from build123d import *
from OCP.BRepFilletAPI import BRepFilletAPI_MakeChamfer

# Parameters (mm, degrees)
SKETCH1_W           = 2.1
SKETCH1_H           = 6.25
BOSS_EXTRUDE1_DEPTH = 39
DRAFT1_ANGLE        = -30
DRAFT2_ANGLE        = -30
CHAMFER1_SIZE       = 0.1
CHAMFER2_SIZE       = 0.273205081
CHAMFER2_SIZE_2     = 0.1
CHAMFER2_SIZE_3     = 0.073205081
CHAMFER2_SIZE_4     = 0.077581461
CHAMFER2_SIZE_5     = 0.171862365


with BuildPart() as part:
    # Sketch1 → Boss-Extrude1 (new, symmetric)
    with BuildSketch(Plane.XY):
        Rectangle(SKETCH1_W, SKETCH1_H)
    extrude(amount=BOSS_EXTRUDE1_DEPTH, both=True)

    # Draft1
    draft1_faces = [part.faces().sort_by_distance(p)[0] for p in [
        (0, 0, 39),
    ]]
    draft(draft1_faces, Plane(origin=(-1.05, 3.125, 39), x_dir=(0, 0, 1), z_dir=(0, 1, 0)), DRAFT1_ANGLE)

    # Draft2
    draft2_faces = [part.faces().sort_by_distance(p)[0] for p in [
        (0, 0, -39),
    ]]
    draft(draft2_faces, Plane(origin=(-1.05, 3.125, 39), x_dir=(0, 0, 1), z_dir=(0, 1, 0)), DRAFT2_ANGLE)

    # Chamfer1
    chamfer1_edges = [part.edges().sort_by_distance(p)[0] for p in [
        (1.05, -3.125, 0),
        (-1.05, -3.125, 0),
        (-1.05, 3.125, 0),
        (1.05, 3.125, 0),
    ]]
    chamfer(chamfer1_edges, length=CHAMFER1_SIZE)

    # Chamfer2
    chamfer2_edges_1 = [part.edges().sort_by_distance(p)[0] for p in [
        (0, -3.125, -35.391560818),
    ]]
    chamfer2_side_1 = [part.faces().sort_by_distance(p)[0] for p in [
        (0, -3.125, -35.389560818),
    ]]
    chamfer2_edges_2 = [part.edges().sort_by_distance(p)[0] for p in [
        (0, -3.125, 35.391560818),
    ]]
    chamfer2_side_2 = [part.faces().sort_by_distance(p)[0] for p in [
        (0, -3.125, 35.389560818),
    ]]
    chamfer2_edges_3 = [part.edges().sort_by_distance(p)[0] for p in [
        (0, 3.125, -39),
    ]]
    chamfer2_side_3 = [part.faces().sort_by_distance(p)[0] for p in [
        (0, 3.123732051, -38.999267949),
    ]]
    chamfer2_edges_4 = [part.edges().sort_by_distance(p)[0] for p in [
        (1, 3.075, -38.971132487),
    ]]
    chamfer2_side_4 = [part.faces().sort_by_distance(p)[0] for p in [
        (0.998827079, 3.074120309, -38.970624597),
    ]]
    chamfer2_edges_5 = [part.edges().sort_by_distance(p)[0] for p in [
        (1, 3.075, 38.971132487),
    ]]
    chamfer2_side_5 = [part.faces().sort_by_distance(p)[0] for p in [
        (0.998827079, 3.074120309, 38.970624597),
    ]]
    chamfer2_edges_6 = [part.edges().sort_by_distance(p)[0] for p in [
        (-1, 3.075, -38.971132487),
    ]]
    chamfer2_side_6 = [part.faces().sort_by_distance(p)[0] for p in [
        (-0.998827079, 3.074120309, -38.970624597),
    ]]
    chamfer2_edges_7 = [part.edges().sort_by_distance(p)[0] for p in [
        (-1, 3.075, 38.971132487),
    ]]
    chamfer2_side_7 = [part.faces().sort_by_distance(p)[0] for p in [
        (-0.998827079, 3.074120309, 38.970624597),
    ]]
    chamfer2_edges_8 = [part.edges().sort_by_distance(p)[0] for p in [
        (0, 3.125, 39),
    ]]
    chamfer2_side_8 = [part.faces().sort_by_distance(p)[0] for p in [
        (0, 3.123732051, 38.999267949),
    ]]
    chamfer2 = BRepFilletAPI_MakeChamfer(part.part.solid().wrapped)
    for e in chamfer2_edges_1:
        chamfer2.Add(CHAMFER2_SIZE, CHAMFER2_SIZE_2, e.wrapped, chamfer2_side_1[0].wrapped)
    for e in chamfer2_edges_2:
        chamfer2.Add(CHAMFER2_SIZE_2, CHAMFER2_SIZE, e.wrapped, chamfer2_side_2[0].wrapped)
    for e in chamfer2_edges_3:
        chamfer2.Add(CHAMFER2_SIZE_2, CHAMFER2_SIZE_3, e.wrapped, chamfer2_side_3[0].wrapped)
    for e in chamfer2_edges_4:
        chamfer2.Add(CHAMFER2_SIZE_4, CHAMFER2_SIZE_2, e.wrapped, chamfer2_side_4[0].wrapped)
    for e in chamfer2_edges_5:
        chamfer2.Add(CHAMFER2_SIZE_4, CHAMFER2_SIZE_2, e.wrapped, chamfer2_side_5[0].wrapped)
    for e in chamfer2_edges_6:
        chamfer2.Add(CHAMFER2_SIZE_4, CHAMFER2_SIZE_2, e.wrapped, chamfer2_side_6[0].wrapped)
    for e in chamfer2_edges_7:
        chamfer2.Add(CHAMFER2_SIZE_4, CHAMFER2_SIZE_2, e.wrapped, chamfer2_side_7[0].wrapped)
    for e in chamfer2_edges_8:
        chamfer2.Add(CHAMFER2_SIZE_3, CHAMFER2_SIZE_2, e.wrapped, chamfer2_side_8[0].wrapped)
    add(Compound.cast(chamfer2.Shape()), mode=Mode.REPLACE)
    chamfer2_2_edges_1 = [part.edges().sort_by_distance(p)[0] for p in [
        (1.04330127, -3.03169873, -35.445428331),
    ]]
    chamfer2_2_side_1 = [part.faces().sort_by_distance(p)[0] for p in [
        (1.043835793, -3.031164207, -35.443576691),
    ]]
    chamfer2_2_edges_2 = [part.edges().sort_by_distance(p)[0] for p in [
        (-1.04330127, -3.03169873, -35.445428331),
    ]]
    chamfer2_2_side_2 = [part.faces().sort_by_distance(p)[0] for p in [
        (-1.043835793, -3.031164207, -35.443576691),
    ]]
    chamfer2_2 = BRepFilletAPI_MakeChamfer(part.part.solid().wrapped)
    for e in chamfer2_2_edges_1:
        chamfer2_2.Add(CHAMFER2_SIZE_2, CHAMFER2_SIZE_5, e.wrapped, chamfer2_2_side_1[0].wrapped)
    for e in chamfer2_2_edges_2:
        chamfer2_2.Add(CHAMFER2_SIZE_2, CHAMFER2_SIZE_5, e.wrapped, chamfer2_2_side_2[0].wrapped)
    add(Compound.cast(chamfer2_2.Shape()), mode=Mode.REPLACE)
    chamfer2_3_edges = [part.edges().sort_by_distance(p)[0] for p in [
        (1.05, 0.062360956, -37.231784524),
        (-1.05, 0.062360956, -37.231784524),
        (-1.05, 0.016985957, 37.205587256),
        (1.05, 0.016985957, 37.205587256),
    ]]
    chamfer(chamfer2_3_edges, length=CHAMFER2_SIZE_2)


solid = part.part
Read the model definition and answer for the solid it produces. Units are mm, in the model's axes. Coordinates: 2 decimals unless noted, no trailing zeros. Loops run counter-clockwise (first coordinate to the right, second up) from the corner with the lowest first, then second, coordinate; pieces in that order, holes last. Notation, with made-up numbers: (63.5, 8.25) -> (116.5, 8.25) arc R12 ccw to (116.5, 26.25) -> close; hole circle Ø9 at (70.5, 40). An arc over 180 degrees is marked (long way). Answer in a Markdown table with one row per item.
Item 1: Straight lines are drawn through the part: line 1 along Z through (x, y) = (0.05, 2); line 2 along Z through (x, y) = (0.05, 1.5). For each, find the intervals that lie inside material, in ascending order. Write a range as [from, to].
Returned:
| item | result |
|---|---|
| line 1 | z = [-38.35, 38.35] |
| line 2 | z = [-38.06, 38.06] |
Item 2: A cutting plane is placed at B-B on y = -1.25. Determine the outline of the cut face in (x, z), plus the area to 3 significant figures.
Returned:
| item | result |
|---|---|
| outline | (-1.05, -36.36) -> (-0.95, -36.47) -> (0.95, -36.47) -> (1.05, -36.36) -> (1.05, 36.36) -> (0.95, 36.47) -> (-0.95, 36.47) -> (-1.05, 36.36) -> close |
| area | 153 mm^2 |
Item 3: A cutting plane is placed at A-A on y = 1.5. Determine the outline of the cut face in (x, z).
Returned:
| item | result |
|---|---|
| outline | (-1.05, -37.95) -> (-0.95, -38.06) -> (0.95, -38.06) -> (1.05, -37.95) -> (1.05, 37.95) -> (0.95, 38.06) -> (-0.95, 38.06) -> (-1.05, 37.95) -> close |
